from build123d import *

# Parameters (mm, degrees)
F0_W     = 254
F0_H     = 40
F1_DEPTH = 4.7625
F2_R     = 2.6
F3_DEPTH = 25.4
F4_W     = 4.7625
F4_H     = 5
F5_DEPTH = 25.4
F6_R     = 1.1
F7_DEPTH = 25.4


with BuildPart() as f1:
    # F0 (on Top) → F1 (new body)
    with BuildSketch(Plane.XY):
        Rectangle(F0_W, F0_H)
    extrude(amount=F1_DEPTH)

    # F2 (on face) → F3 (cut)
    with BuildSketch(Plane.XY.offset(4.7625)):
        with Locations((-96, -4.5)):
            Circle(F2_R)
        with Locations((-85, -4.5)):
            Circle(F2_R)
        with Locations((-74, -4.5)):
            Circle(F2_R)
        with Locations((-63, -4.5)):
            Circle(F2_R)
        with Locations((-52, -4.5)):
            Circle(F2_R)
        with Locations((-41, -4.5)):
            Circle(F2_R)
        with Locations((-30, -4.5)):
            Circle(F2_R)
        with Locations((-19, -4.5)):
            Circle(F2_R)
        with Locations((-8, -4.5)):
            Circle(F2_R)
        with Locations((3, -4.5)):
            Circle(F2_R)
        with Locations((14, -4.5)):
            Circle(F2_R)
        with Locations((25, -4.5)):
            Circle(F2_R)
        with Locations((36, -4.5)):
            Circle(F2_R)
        with Locations((47, -4.5)):
            Circle(F2_R)
        with Locations((58, -4.5)):
            Circle(F2_R)
        with Locations((69, -4.5)):
            Circle(F2_R)
        with Locations((80, -4.5)):
            Circle(F2_R)
        with Locations((-90.5, 15.5)):
            Circle(F2_R)
        with Locations((-79.5, 15.5)):
            Circle(F2_R)
        with Locations((-68.5, 15.5)):
            Circle(F2_R)
        with Locations((-57.5, 15.5)):
            Circle(F2_R)
        with Locations((-46.5, 15.5)):
            Circle(F2_R)
        with Locations((-35.5, 15.5)):
            Circle(F2_R)
        with Locations((-24.5, 15.5)):
            Circle(F2_R)
        with Locations((-13.5, 15.5)):
            Circle(F2_R)
        with Locations((-2.5, 15.5)):
            Circle(F2_R)
        with Locations((8.5, 15.5)):
            Circle(F2_R)
        with Locations((19.5, 15.5)):
            Circle(F2_R)
        with Locations((30.5, 15.5)):
            Circle(F2_R)
        with Locations((41.5, 15.5)):
            Circle(F2_R)
        with Locations((52.5, 15.5)):
            Circle(F2_R)
        with Locations((63.5, 15.5)):
            Circle(F2_R)
        with Locations((74.5, 15.5)):
            Circle(F2_R)
        with Locations((93, -8.5)):
            Circle(F2_R)
    extrude(amount=-F3_DEPTH, mode=Mode.SUBTRACT)

    # F4 (on face) → F5 (cut)
    with BuildSketch(Plane.XY.offset(4.7625)):
        with Locations((-124.61875, 17.5)):
            Rectangle(F4_W, F4_H)
        Polygon((-127, 5), (-127, 0), (-127, -5), (-122.2375, -5), (-122.2375, 0), (-122.2375, 5), align=None)
        with Locations((-124.61875, -17.5)):
            Rectangle(F4_W, F4_H)
        with Locations((124.61875, 17.5)):
            Rectangle(F4_W, F4_H)
        Polygon((127, -5), (127, 0), (127, 5), (122.2375, 5), (122.2375, 0), (122.2375, -5), align=None)
        with Locations((124.61875, -17.5)):
            Rectangle(F4_W, F4_H)
    extrude(amount=-F5_DEPTH, mode=Mode.SUBTRACT)

    # F6 (on face) → F7 (cut)
    with BuildSketch(Plane.XY.offset(4.7625)):
        with Locations((124.61875, 10)):
            Circle(F6_R)
        with Locations((124.61875, -10)):
            Circle(F6_R)
        with Locations((-124.61875, -10)):
            Circle(F6_R)
        with Locations((-124.61875, 10)):
            Circle(F6_R)
    extrude(amount=-F7_DEPTH, mode=Mode.SUBTRACT)


solid = f1.part
The listing builds one solid part. Answer for the finished solid, in the listing's coordinates (mm). A direction names the side the tool comes from. Give positions to 0.01 mm unless a question says otherwise; leave off trailing zeros. Write each loop counter-clockwise with the first axis right and the second up, starting at its lowest first coordinate (ties: lowest second). Pieces come first, ordered by that corner, then holes.
1) Section B-B (z = 2.9) is taken. Count the separate pieces of the cut face and the enclosed holes in it, and give its area (3 significant figures).
2) For a pull along Y with two mould halves and no side action, classify faces 1 (the face through (49.9, 15.6, 2.4)), 2 (the face through (-65.6, -4.4, 2.4)), 3 (the face through (-125, 15, 2)), 4 (the face through (-127, -10, 2)) as pulls with the +Y half, pulls with the -Y half, needs draft (parallel to the pull), parting line crosses it, or undercut.
3) Find the intervals of material crossed by L1, parallel to X at y = 11, z = 1.8; L2, parallel to Y at x = 36, z = 1.6; L3, parallel to Y at x = -24.5, z = 3.5, in increasing order.
4) Section A-A (x = 14) is taken. Write down the section's boundary in (y, z).
5) Given P1, Ø1.4, axis at x = -124, z = 3.5, coming from the +Y side, flat-ended and moving along its own axis, determine where the tip first touches the part or whether it passes through.
6) A tool of negligible diameter and unlimited length cuts with its end or side. For faces 5 (the face through (-125, 5, 2)), 6 (the face through (-122.238, 17, 2)), 7 (the face through (-16.6, -5.5, 2.4)), from which of +Z, -Z, +X, -X, +Y, -Y can it reach the whole face along a straight path? Write none if from no direction.
Response:
1. separate pieces: 1
1. enclosed holes: 38
1. area: 9,230 mm2
2. face 1: undercut
2. face 2: undercut
2. face 3: pulls with the +Y half
2. face 4: needs draft
3. L1: x = -127 to -125.08, -124.16 to 124.16, 125.08 to 127
3. L2: y = -20 to -7.1, -1.9 to 20
3. L3: y = -20 to 12.9, 18.1 to 20
4. outline: (-20, 0) - (-7.1, 0) - (-7.1, 4.76) - (-20, 4.76) - close; (-1.9, 0) - (20, 0) - (20, 4.76) - (-1.9, 4.76) - close
5. P1: stops at y = 15
6. face 5: +Z, -Z, -X
6. face 6: +Z, -Z, -X, +Y
6. face 7: +Z, -Z
